Here's the drawing with two shaded views (mm, measured from the low corner). I have some questions. A direction names the side the tool comes from. Coordinates: 2 decimals unless noted, no trailing zeros. Write each loop counter-clockwise with the first axis right and the second up, starting at its lowest first coordinate (ties: lowest second). Pieces come first, ordered by that corner, then holes. Notation, with made-up numbers: (28, 15.5) -> (66, 15.5) arc R16 cw to (66, 43.5) -> close; hole circle Ø8 at (-22, 61.5). An arc over 180 degrees is marked (long way). Put each result on its own line as item: value.
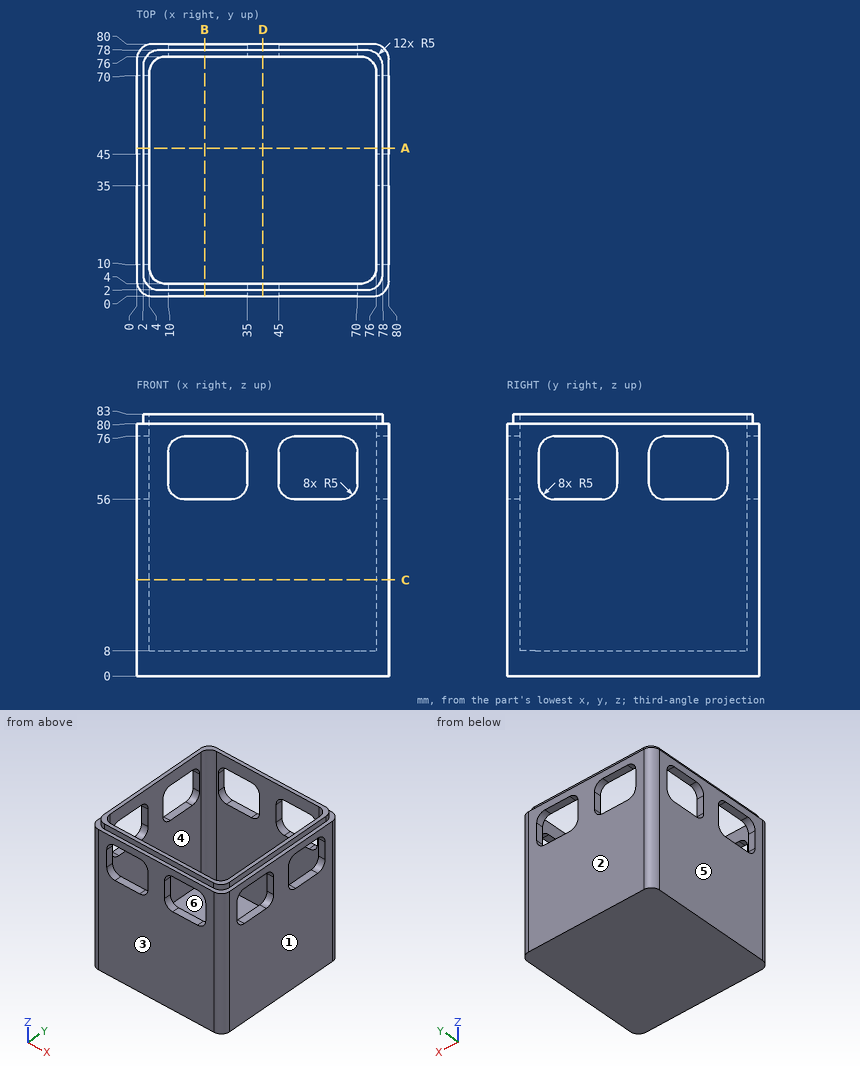
Item 1: Imagine slicing it at D-D on x = 40. Write out the boundary of the cut face in (y, z).
Output:
outline: (0, 0) -> (80, 0) -> (80, 80) -> (78, 80) -> (78, 83) -> (76, 83) -> (76, 8) -> (4, 8) -> (4, 83) -> (2, 83) -> (2, 80) -> (0, 80) -> close
Item 2: For P1, Ø1.5, axis at x = 54, z = 82, coming from the -Y side; P2, Ø1.2, axis at y = 77, z = 66.5, coming from the -X side; P3, Ø0.9, axis at x = 50.5, z = 81.5, coming from the +Y side, each with a flat end and sliding along its axis, tell me the tip position at first contact or that it passes through.
Output:
P1: stops at y = 2
P2: stops at x = 0.2
P3: stops at y = 78
Item 3: Please list where these lines run through material, in increasing order: line 1 along Y through (x, z) = (68.5, 27.5); line 2 along Z through (x, y) = (36, 53.5). Write a range as from..to.
Output:
line 1: y = 0..4, 76..80
line 2: z = 0..8
Item 4: Imagine slicing it at A-A on y = 47. Write out the boundary of the cut face in (x, z), then the cut area to 3 significant figures.
Output:
outline: (0, 0) -> (80, 0) -> (80, 57) -> (76, 57) -> (76, 8) -> (4, 8) -> (4, 57) -> (0, 57) -> close; (0, 75) -> (4, 75) -> (4, 83) -> (2, 83) -> (2, 80) -> (0, 80) -> close; (76, 75) -> (80, 75) -> (80, 80) -> (78, 80) -> (78, 83) -> (76, 83) -> close
area: 1,080 mm²
Item 5: Imagine slicing it at C-C on z = 30.5. Write out the boundary of the cut face in (x, y).
Output:
outline: (0, 5) arc R5 ccw to (5, 0) -> (75, 0) arc R5 ccw to (80, 5) -> (80, 75) arc R5 ccw to (75, 80) -> (5, 80) arc R5 ccw to (0, 75) -> close; hole (4, 9) arc R5 ccw to (9, 4) -> (71, 4) arc R5 ccw to (76, 9) -> (76, 71) arc R5 ccw to (71, 76) -> (9, 76) arc R5 ccw to (4, 71) -> close
Item 6: If we mould it in two halves opening along Y, with no side actions, what happens to the marked faces 1, 2, 3 and 4? For each: released by +Y, released by -Y, zero draft, split by the parting line, or undercut.
Output:
face 1: zero draft
face 2: released by +Y
face 3: released by -Y
face 4: undercut
Item 7: Which directions (+Z, -Z, +X, -X, +Y, -Y) give clear straight access to the entire face, cutting with the end or side of a thin tool? Please do the marked faces 5 and 6.
Output:
face 5: +Z, -Z, -X, +Y, -Y
face 6: +Z
Item 8: Imagine slicing it at B-B on x = 21.5. Write out the boundary of the cut face in (y, z), then the cut area to 3 significant figures.
Output:
outline: (0, 0) -> (80, 0) -> (80, 56) -> (76, 56) -> (76, 8) -> (4, 8) -> (4, 56) -> (0, 56) -> close; (0, 76) -> (4, 76) -> (4, 83) -> (2, 83) -> (2, 80) -> (0, 80) -> close; (76, 76) -> (80, 76) -> (80, 80) -> (78, 80) -> (78, 83) -> (76, 83) -> close
area: 1,070 mm²
